```python
from build123d import *

# Parameters (mm, degrees)
SKETCH_1_R               = 19
EXTRUDE_1_DEPTH          = 10
SKETCH_2_R               = 8
CUT_EXTRUDE_1_DEPTH      = 2
SKETCH_3_R               = 6
CUT_EXTRUDE_2_DEPTH      = 3
SKETCH_4_R               = 2.5
CUT_EXTRUDE_3_DEPTH      = 16
SKETCH_5_R               = 4
CUT_EXTRUDE_4_DEPTH      = 4.4
SKETCH_6_R               = 2.5
CUT_EXTRUDE_5_DEPTH      = 28.447404249
PATTERN_CIRCULAR_1_COUNT = 4


with BuildPart() as part:
    # 草图1 → 凸台-拉伸1 (new body)
    with BuildSketch(Plane(origin=(0, 0, 0), x_dir=(1, 0, 0), z_dir=(0, 1, 0))):
        with Locations(Location((0, 0, 0), (0, 0, 270))):
            Circle(SKETCH_1_R)
    extrude(amount=EXTRUDE_1_DEPTH)

    # 草图2 → 切除-拉伸1 (cut)
    with BuildSketch(Plane(origin=(0, 10, 0), x_dir=(1, 0, 0), z_dir=(0, 1, 0))):
        with Locations(Location((0, 0, 0), (0, 0, 270))):
            Circle(SKETCH_2_R)
    extrude(amount=-CUT_EXTRUDE_1_DEPTH, mode=Mode.SUBTRACT)

    # 草图3 → 切除-拉伸2 (cut)
    with BuildSketch(Plane.XZ):
        with Locations(Location((0, 0, 0), (0, 0, 270))):
            Circle(SKETCH_3_R)
    extrude(amount=-CUT_EXTRUDE_2_DEPTH, mode=Mode.SUBTRACT)

    # 草图4 → 切除-拉伸3 (cut)
    with BuildSketch(Plane.XZ.offset(-3)):
        with Locations(Location((0, 0, 0), (0, 0, 270))):
            Circle(SKETCH_4_R)
    extrude(amount=-CUT_EXTRUDE_3_DEPTH, mode=Mode.SUBTRACT)

    # 草图5 → 切除-拉伸4 (cut)
    with BuildSketch(Plane(origin=(0, 10, 0), x_dir=(1, 0, 0), z_dir=(0, 1, 0))):
        with Locations(Location((0, 14, 0), (0, 0, 270))):
            Circle(SKETCH_5_R)
    cut_extrude_4 = extrude(amount=-CUT_EXTRUDE_4_DEPTH, mode=Mode.SUBTRACT)

    # 草图6 → 切除-拉伸5 (cut, through all)
    with BuildSketch(Plane(origin=(0, 5.6, 0), x_dir=(1, 0, 0), z_dir=(0, 1, 0))):
        with Locations(Location((0, 14, 0), (0, 0, 270))):
            Circle(SKETCH_6_R)
    cut_extrude_5 = extrude(amount=-CUT_EXTRUDE_5_DEPTH, mode=Mode.SUBTRACT)

    # 阵列(圆周)1: 切除-拉伸4, 切除-拉伸5 ×4 about axis
    pattern_circular_1_axis = Axis((0, 0, 0), (0, 1, 0))
    add([cut_extrude_4.rotate(pattern_circular_1_axis, i * 360 / PATTERN_CIRCULAR_1_COUNT) for i in range(1, PATTERN_CIRCULAR_1_COUNT)], mode=Mode.SUBTRACT)
    add([cut_extrude_5.rotate(pattern_circular_1_axis, i * 360 / PATTERN_CIRCULAR_1_COUNT) for i in range(1, PATTERN_CIRCULAR_1_COUNT)], mode=Mode.SUBTRACT)


solid = part.part
```
Verification items for the finished model (mm, model axes). A direction names the side the tool comes from. Coordinates: 2 decimals unless noted, no trailing zeros. Write each loop counter-clockwise with the first axis right and the second up, starting at its lowest first coordinate (ties: lowest second). Pieces come first, ordered by that corner, then holes. Notation, with made-up numbers: M -3.5,-19.75 L 4.5,-19.75 A26 ccw 4.5,6.25 Z; hole C 43.25,-2.75 d6. An arc over 180 degrees is marked long. One line per item, written item: value.
Item 1: Section check C-C, the plane y = 4.25. Record the boundary of the cut face in (x, z).
Check sheet entries:
outline: C 0,0 d38; hole C -14,0 d5; hole C 0,-14 d5; hole C 0,0 d5; hole C 0,14 d5; hole C 14,0 d5
Item 2: Access from +Z, -Z, +X, -X, +Y, -Y to the whole of each face (thin tool, end or side, straight path). Record for faces 4 (the flat face through (0, 3, -3)), 5 (the flat face through (4.5, 0, -4.5)), 6 (the flat face through (-16, 5.6, 2)).
Check sheet entries:
face 4: -Y
face 5: +Z, -Z, +X, -X, -Y
face 6: +Y
Item 3: Mould release check, pull along X, two halves, no side actions. Record for faces 1 (the cylindrical face through (-7.81, 9.01, -1.73)), 2 (the flat face through (0.3, 10, 8.2)), 3 (the cylindrical face through (-11.56, 4.93, -15.08)): pulls with the +X half, pulls with the -X half, needs draft (parallel to the pull), parting line crosses it, or undercut.
Check sheet entries:
face 1: undercut
face 2: needs draft
face 3: parting line crosses it
Item 4: Gauge pin test, flat ends, axial feed: pin 1 Ø4.5 at (x, z) = (14, 0) entering from +Y; pin 2 Ø1.5 at (x, y) = (7.5, 6.5) entering from -Z; pin 3 Ø4 at (x, y) = (8, 3) entering from +Z; pin 4 Ø6 at (y, z) = (8, -2) entering from -X. Record the tip position at first contact, or that the pin passes through.
Check sheet entries:
pin 1: passes through
pin 2: stops at z = -17.76
pin 3: stops at z = 18.03
pin 4: stops at x = -19
Item 5: Section check A-A, the plane x = 0. State how many separate pieces and enclosed holes the cut face has, plus the area to 3 significant figures.
Check sheet entries:
separate pieces: 4
enclosed holes: 0
area: 161 mm^2
Item 6: Section check D-D, the plane x = 13.5. Record the boundary of the cut face in (y, z), plus the area to 3 significant figures.
Check sheet entries:
outline: M 0,-13.37 L 10,-13.37 L 10,-3.97 L 5.6,-3.97 L 5.6,-2.45 L 0,-2.45 Z; M 0,2.45 L 5.6,2.45 L 5.6,3.97 L 10,3.97 L 10,13.37 L 0,13.37 Z
area: 205 mm^2
Item 7: Scan lines: line 1 along Z through (x, y) = (-0.5, 6.25); line 2 along X through (y, z) = (6.75, -2); line 3 along Z through (x, y) = (0.5, 3.5). Record each from-to range of solid material in increasing order.
Check sheet entries:
line 1: z = -18.99 to -17.97, -10.03 to -2.45, 2.45 to 10.03, 17.97 to 18.99
line 2: x = -18.89 to -17.46, -10.54 to -1.5, 1.5 to 10.54, 17.46 to 18.89
line 3: z = -18.99 to -16.45, -11.55 to -2.45, 2.45 to 11.55, 16.45 to 18.99
